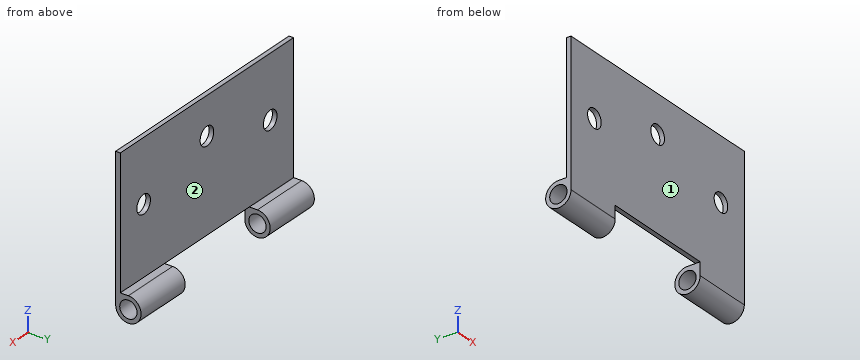
Autodesk Inventor part; units mm, degrees
ref_plane "YZ Plane" through (0, 0, 0) normal (1, 0, 0) x (0, 1, 0)
ref_plane "XZ Plane" through (0, 0, 0) normal (0, 1, 0) x (-1, 0, 0)
ref_plane "XY Plane" through (0, 0, 0) normal (0, 0, 1) x (1, 0, 0)
sketch "Boceto1" plane through (0, 0, 0) normal (0, 1, 0) x (-1, 0, 0)
  line L0 (11.708, 26.8389) -> (11.708, -1.1611)
  line L1 (11.708, -1.1611) -> (-39.292, -1.1611)
  line L2 (-39.292, -1.1611) -> (-39.292, 26.8389)
  line L3 (-39.292, 26.8389) -> (11.708, 26.8389)
  circle A0 centre (4.833, 13.4639) radius 2
  circle A1 centre (-32.417, 13.4639) radius 2
  circle A2 centre (-13.792, 18.6686) radius 2
  point P0 (0, 0)
  dimension "d0" = 28
  dimension "d1" = 51
  dimension "d2" = 4
  dimension "d3" = 4
  dimension "d4" = 4
  dimension "d5" = 25.5
  dimension "d6" = 6.875
  dimension "d7" = 13.375
  dimension "d8" = 6.875
  dimension "d9" = 13.375
extrude "Extrusión1" add sketch "Boceto1" along normal blind 1
sketch "Boceto2" plane through (39.292, 0, 26.8389) normal (1, 0, 0) x (0, 0, -1)
  arc A0 (30.75, 0) -> (28, 2.75) centre (30.75, 2.75) ccw
  circle A1 centre (30.75, 2.75) radius 1.875
  line L0 (0, 0) -> (28, 0)
  line L1 (28, 0) -> (28, 1)
  line L2 (28, 0) -> (28, 2.75)
  line L3 (28, 0) -> (30.75, 0)
  point P0 (26.8389, 0)
  dimension "d12" = 5.5
  dimension "d13" = 3.75
extrude "Extrusión2" add sketch "Boceto2" against normal blind 51
sketch "Boceto3" plane through (0, 0, 0) normal (0, -1, 0) x (1, 0, 0)
  line L0 (39.292, -1.1611) -> (-11.708, -1.1611)
  line L1 (39.292, -1.1611) -> (-11.708, -1.1611)
  line L2 (-11.708, -2.0361) -> (39.292, -2.0361)
  line L3 (13.792, -1.1611) -> (26.292, -1.1611)
  line L4 (26.292, -1.1611) -> (1.292, -1.1611)
  line L5 (1.292, -1.1611) -> (1.292, -7.7765)
  line L6 (1.292, -7.7765) -> (26.292, -7.7765)
  line L7 (26.292, -7.7765) -> (26.292, -1.1611)
  dimension "d16" = 12.5
  dimension "d17" = 25
extrude "Extrusión3" cut sketch "Boceto3" against normal blind 51
properties part number "Ala 1 Bisagra tipo Libro Grande"
Can you work these out from the model? Positions are in its coordinate system, mm. Face numbers are marked on the shaded views. A direction names the side the tool comes from. Coordinates: 2 decimals unless noted, no trailing zeros. Write each loop counter-clockwise with the first axis right and the second up, starting at its lowest first coordinate (ties: lowest second). Pieces come first, ordered by that corner, then holes. Notation, with made-up numbers: (31.5, 75) -> (37.5, 75) arc R31 ccw to (37.5, 111) -> close; hole circle Ø3 at (15.25, 88). An arc over 180 degrees is marked (long way). Answer as CSV lines item,"result".
1) On a 3-axis mill with a long thin cutter (end or side, diameter ignored), from which of +Z, -Z, +X, -X, +Y, -Y can I reach the whole of each face in a straight line? I mean the marked faces 1 and 2. Say none if no direction works.
Check result:
face 1,"+Z, -Z, +X, -X, -Y"
face 2,"+Z, +X, -X, +Y"
2) If I drill on line 1 (Y direction, x = 0.5, z = 0); line 2 (Z direction, x = -3, y = 2.3); line 3 (Z direction, x = 30, y = 1.95), over which ranges is the centre line in solid material (lowest first)? Write a range as from..to.
Check result:
line 1,"0..1"
line 2,"-6.62..-5.73, -2.09..-1.16"
line 3,"-6.54..-5.61, -2.22..-1.16"
3) Will these pins go through, and if not, where does the flat tip stop? P1, Ø3, axis at x = 25.5, y = 4.5, coming from the +Z side; P2, Ø1.5, axis at x = 18, y = 2, coming from the -Z side; P3, Ø5, axis at x = 13.79, z = 18.67, coming from the +Y side; P4, Ø1, axis at x = -4, y = 1.5, coming from the -Z side.
Check result:
P1,"z = -1.2"
P2,"through"
P3,"y = 1"
P4,"z = -6.56"
4) If we section it at A-A on x = 13.5: Please give me the cut outline in (y, z).
Check result:
outline,"(0, -1.16) -> (1, -1.16) -> (1, 16.69) -> (0, 16.69) -> close; (0, 20.65) -> (1, 20.65) -> (1, 26.84) -> (0, 26.84) -> close"
5) If we section it at B-B on z = 5.5: Please give me the cut outline in (x, y).
Check result:
outline,"(-11.71, 0) -> (39.29, 0) -> (39.29, 1) -> (-11.71, 1) -> close"
6) If we section it at C-C on x = 22.5: Please give me the cut outline in (y, z).
Check result:
outline,"(0, -1.16) -> (1, -1.16) -> (1, 26.84) -> (0, 26.84) -> close"
